Design review of the part built by this model. Coordinates are the model's own, in mm. A direction names the side the tool comes from. Round coordinates to 2 decimals unless told otherwise and drop trailing zeros. Loops run counter-clockwise (first coordinate to the right, second up) from the corner with the lowest first, then second, coordinate; pieces in that order, holes last. Notation, with made-up numbers: (51.25, 55.5) -> (107.25, 55.5) arc R24 ccw to (107.25, 88.5) -> close; hole circle Ø11 at (82, 18.25). An arc over 180 degrees is marked (long way). Answer as CSV lines item,"result". Start each with the question number.
```python
from build123d import *

# Parameters (mm, degrees)
EXTRUDE_1_DEPTH     = 50
SKETCH_2_W          = 42
SKETCH_2_H          = 25
CUT_EXTRUDE_1_DEPTH = 37
SKETCH_3_R          = 2.5
CUT_EXTRUDE_2_DEPTH = 37
SKETCH_4_R          = 5
CUT_EXTRUDE_3_DEPTH = 147
SKETCH_5_R          = 1.5
CUT_EXTRUDE_4_DEPTH = 5
SKETCH_6_R          = 1.5
CUT_EXTRUDE_5_DEPTH = 37


with BuildPart() as part:
    # 草图1 → 凸台-拉伸1 (new body)
    with BuildSketch(Plane.XY):
        Polygon((90, 0), (90, 4), (56, 4), (56, 36), (-56, 36), (-56, 4), (-90, 4), (-90, 0), (-50, 0), (-50, 32), (50, 32), (50, 0), align=None)
    extrude(amount=-EXTRUDE_1_DEPTH)

    # 草图2 → 切除-拉伸1 (cut, through all)
    with BuildSketch(Plane(origin=(0, 36, 0), x_dir=(1, 0, 0), z_dir=(0, 1, 0))):
        with Locations((0, 25)):
            Rectangle(SKETCH_2_W, SKETCH_2_H)
    extrude(amount=-CUT_EXTRUDE_1_DEPTH, mode=Mode.SUBTRACT)

    # 草图3 → 切除-拉伸2 (cut, through all)
    with BuildSketch(Plane(origin=(0, 36, 0), x_dir=(1, 0, 0), z_dir=(0, 1, 0))):
        with Locations((-24.76, 30)):
            Circle(SKETCH_3_R)
        with Locations((24.76, 30)):
            Circle(SKETCH_3_R)
        with Locations((24.76, 20)):
            Circle(SKETCH_3_R)
        with Locations((-24.76, 20)):
            Circle(SKETCH_3_R)
    extrude(amount=-CUT_EXTRUDE_2_DEPTH, mode=Mode.SUBTRACT)

    # 草图4 → 切除-拉伸3 (cut, through all)
    with BuildSketch(Plane(origin=(56, 0, 0), x_dir=(0, 0, -1), z_dir=(1, 0, 0))):
        with Locations((25, 11)):
            Circle(SKETCH_4_R)
    extrude(amount=-CUT_EXTRUDE_3_DEPTH, mode=Mode.SUBTRACT)

    # 草图5 → 切除-拉伸4 (cut, through all)
    with BuildSketch(Plane(origin=(0, 4, 0), x_dir=(1, 0, 0), z_dir=(0, 1, 0))):
        with Locations((-36.607969405, 54.749619062)):
            Circle(SKETCH_5_R)
        with Locations((-65, 42.286041433)):
            Circle(SKETCH_5_R)
        with Locations((-65, 7.713958567)):
            Circle(SKETCH_5_R)
        with Locations((-36.607969405, -4.749619062)):
            Circle(SKETCH_5_R)
        with Locations((36.607969405, -4.749619062)):
            Circle(SKETCH_5_R)
        with Locations((65, 7.713958567)):
            Circle(SKETCH_5_R)
        with Locations((65, 42.286041433)):
            Circle(SKETCH_5_R)
        with Locations((36.607969405, 54.749619062)):
            Circle(SKETCH_5_R)
        with Locations((85, 7.713958567)):
            Circle(SKETCH_5_R)
        with Locations((85, 42.286041433)):
            Circle(SKETCH_5_R)
        with Locations((-85, 42.286041433)):
            Circle(SKETCH_5_R)
        with Locations((-85, 7.713958567)):
            Circle(SKETCH_5_R)
    extrude(amount=-CUT_EXTRUDE_4_DEPTH, mode=Mode.SUBTRACT)

    # 草图6 → 切除-拉伸5 (cut, through all)
    with BuildSketch(Plane(origin=(0, 36, 0), x_dir=(1, 0, 0), z_dir=(0, 1, 0))):
        with Locations((-7, 45)):
            Circle(SKETCH_6_R)
        with Locations((7, 45)):
            Circle(SKETCH_6_R)
        with Locations((-15, 45)):
            Circle(SKETCH_6_R)
        with Locations((15, 45)):
            Circle(SKETCH_6_R)
        with Locations((15, 5)):
            Circle(SKETCH_6_R)
        with Locations((7, 5)):
            Circle(SKETCH_6_R)
        with Locations((-7, 5)):
            Circle(SKETCH_6_R)
        with Locations((-15, 5)):
            Circle(SKETCH_6_R)
    extrude(amount=-CUT_EXTRUDE_5_DEPTH, mode=Mode.SUBTRACT)


solid = part.part
```
Q1. To check wall thickness, follow probe 1 along X at (y, z) = (8, -41); probe 2 along Z at (x, y) = (-15, 34); probe 3 along X at (y, z) = (33, -5). State the ranges of each line that lie inside material, in increasing order. Write a range as from..to.
Q2. Mouldability with a two-part tool opening along X and no side actions: class faces 6 (the cylindrical face through (-63.569, 2.028, -8.165)), 7 (the flat face through (-90, 2, -25)), 8 (the flat face through (56, 20, -25)), 9 (the flat face through (1, 36, -41)) as pulls with the +X half, pulls with the -X half, needs draft (parallel to the pull), parting line crosses it, or undercut.
Q3. Add section A-A, the plane x = -24.76. Give the boundary of the cut face in (y, z).
Q4. Add section D-D, the plane x = 41. Give the boundary of the cut face in (y, z).
Q5. For pin 1 Ø3.5 at (x, z) = (7, -45) entering from -Y; pin 2 Ø3.5 at (x, z) = (85, -7.71) entering from +Y; pin 3 Ø4 at (x, z) = (-24.76, -20) entering from +Y; pin 4 Ø3 at (y, z) = (9.5, -21) entering from -X, all flat-tipped, find the tip position at first contact; note any pin that passes through.
Q6. Add section C-C, the plane x = 0.5. Give the boundary of the cut face in (y, z), and give its area (3 significant figures).
Q7. Add section B-B, the plane y = 11. Give the boundary of the cut face in (x, z), and give its area (3 significant figures).
Q8. Machinability: for faces 1 (the flat face through (-56, 20, -25)), 2 (the flat face through (70, 0, -25)), 3 (the flat face through (0, 34, -37.5)), 4 (the cylindrical face through (53, 11, -20)), 5 (the flat face through (-50, 19, -25)), which of the approach directions +Z, -Z, +X, -X, +Y, -Y give a long, thin tool a straight path to every point of the face, cutting with its end or side? Answer none if there is none.
Worked answers:
1,probe 1,"x = -56..-50, 50..56"
1,probe 2,"z = -50..-46.5, -43.5..-37.5, -12.5..-6.5, -3.5..0"
1,probe 3,"x = -56..-16.5, -13.5..-8.5, -5.5..5.5, 8.5..13.5, 16.5..56"
2,face 6,"undercut"
2,face 7,"pulls with the -X half"
2,face 8,"pulls with the +X half"
2,face 9,"needs draft"
3,outline,"(32, -50) -> (36, -50) -> (36, -32.5) -> (32, -32.5) -> close; (32, -27.5) -> (36, -27.5) -> (36, -22.5) -> (32, -22.5) -> close; (32, -17.5) -> (36, -17.5) -> (36, 0) -> (32, 0) -> close"
4,outline,"(32, -50) -> (36, -50) -> (36, 0) -> (32, 0) -> close"
5,pin 1,"stops at y = 32"
5,pin 2,"stops at y = 4"
5,pin 3,"passes through"
5,pin 4,"stops at x = -56"
6,outline,"(32, -50) -> (36, -50) -> (36, -37.5) -> (32, -37.5) -> close; (32, -12.5) -> (36, -12.5) -> (36, 0) -> (32, 0) -> close"
6,area,"100 mm^2"
7,outline,"(-56, -50) -> (-50, -50) -> (-50, -30) -> (-56, -30) -> close; (-56, -20) -> (-50, -20) -> (-50, 0) -> (-56, 0) -> close; (50, -50) -> (56, -50) -> (56, -30) -> (50, -30) -> close; (50, -20) -> (56, -20) -> (56, 0) -> (50, 0) -> close"
7,area,"480 mm^2"
8,face 1,"+Z, -Z, -X, +Y"
8,face 2,"+Z, -Z, +X, -X, -Y"
8,face 3,"+Y, -Y"
8,face 4,"+X, -X"
8,face 5,"+Z, -Z, -Y"
